Could you check a few things on this model? Use its own coordinates, in mm. Face numbers are marked on the shaded views. A direction names the side the tool comes from. Coordinates: 2 decimals unless noted, no trailing zeros. Loops run counter-clockwise (first coordinate to the right, second up) from the corner with the lowest first, then second, coordinate; pieces in that order, holes last. Notation, with made-up numbers: (-39, 62.5) - (18, 62.5) arc R23 cw to (18, 96.5) - close; hole circle Ø3 at (57, 59). An arc over 180 degrees is marked (long way). One line per item, written item: value. Start each with the question number.
(1) If we section it at B-B on z = -16.5: Write out the boundary of the cut face in (x, y), then the cut area to 3 significant figures.
(2) I'm going to push flat-ended pins straight in: P1, Ø6, axis at x = 2.5, y = -6.5, coming from the +Z side; P2, Ø4.5, axis at y = 36.81, z = 0, coming from the +X side; P3, Ø1, axis at x = 5.5, z = -2.5, coming from the -Y side. Where does each tip first touch, or does it pass through?
(3) If we section it at C-C on y = 34: Write out the boundary of the cut face in (x, z), then the cut area to 3 significant figures.
(4) If we section it at A-A on x = 5: Write out the boundary of the cut face in (y, z) (3 decimals).
(5) If I drill on line 1 along X through (y, z) = (24.5, 10.5); line 2 along Z through (x, y) = (7.5, 16.5); line 3 along Y through (x, z) = (7.75, -4), over which ranges is the centre line in solid material (lowest first)? Write a range as from..to.
(6) On a 3-axis mill with a long thin cutter (end or side, diameter ignored), from which of +Z, -Z, +X, -X, +Y, -Y can I reach the whole of each face in a straight line? I mean the marked faces 1 and 2. Say none if no direction works.
(7) If we mould it in two halves opening along Y, with no side actions, what happens to the marked faces 3, 4, 5 and 6? For each: pulls with the +Y half, pulls with the -Y half, needs draft (parallel to the pull), parting line crosses it, or undercut.
```python
from build123d import *

# Parameters (mm, degrees)
FILLET1_R          = 3
SKETCH2_R          = 2
CUT_EXTRUDE1_DEPTH = 2


with BuildPart() as part:
    # Sketch1 → Revolve1 (revolve)
    with BuildSketch(Plane.XY):
        Polygon((0, 40.625), (0, 21.25), (10.625, 21.25), (10.625, 10.625), (11.63, 10.625), (11.63, 22.25), (1, 22.25), (1, 29.25), (1, 35.625), (1, 40.625), align=None)
    revolve(axis=Axis((11.63, 10.625, 0), (-1, 0, 0)))

    # Fillet1
    fillet1_edges = [part.edges().sort_by_distance(p)[0] for p in [
        (11.63, -1, 0),
    ]]
    fillet(fillet1_edges, radius=FILLET1_R)

    # Sketch2 → Cut-Extrude1 (cut)
    with BuildSketch(Plane(origin=(1, 0, 0), x_dir=(0, 0, -1), z_dir=(1, 0, 0))):
        with Locations(Location((0, 36.80872946, 0), (0, 0, 90))):
            Circle(SKETCH2_R)
        with Locations(Location((23.175774878, 24.582890134, 0), (0, 0, 90))):
            Circle(SKETCH2_R)
        with Locations(Location((24.175774878, -1.600839326, 0), (0, 0, 90))):
            Circle(SKETCH2_R)
        with Locations(Location((2, -15.55872946, 0), (0, 0, 90))):
            Circle(SKETCH2_R)
        with Locations(Location((-21.175774878, -3.332890134, 0), (0, 0, 90))):
            Circle(SKETCH2_R)
        with Locations(Location((-22.175774878, 22.850839326, 0), (0, 0, 90))):
            Circle(SKETCH2_R)
    extrude(amount=-CUT_EXTRUDE1_DEPTH, mode=Mode.SUBTRACT)


solid = part.part
```
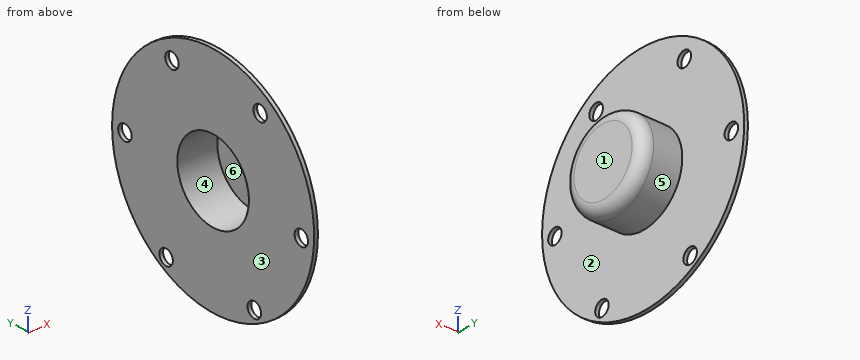
Values:
1. outline: (0, -14.43) - (1, -14.43) - (1, 35.68) - (0, 35.68) - close
1. area: 50.1 mm2
2. P1: stops at z = 26.25
2. P2: stops at x = 1
2. P3: stops at y = -0.83
3. outline: (0, -18.8) - (1, -18.8) - (1, 18.8) - (0, 18.8) - close
3. area: 37.6 mm2
4. outline: circle Ø23.25 at (10.625, 0); hole circle Ø21.25 at (10.625, 0)
5. line 1: x = 0..1
5. line 2: z = -10.03..-8.85, 8.85..10.03
5. line 3: y = -0.29..0.78, 20.47..21.54
6. face 1: +Z, -Z, +X, +Y, -Y
6. face 2: +X
7. face 3: needs draft
7. face 4: undercut
7. face 5: parting line crosses it
7. face 6: undercut
